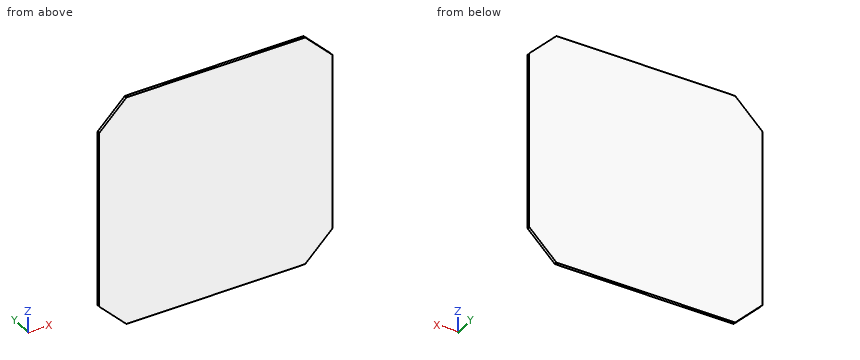
```python
from build123d import *

# Parameters (mm, degrees)
ESBO_O1_W                = 214
ESBO_O1_H                = 214
ESBO_O1_R                = 2.5
RESSALTO_EXTRUS_O1_DEPTH = 1.25
CHANFRO1_SIZE            = 25


with BuildPart() as part:
    # Esboço1 → Ressalto-extrusão1 (new, symmetric)
    with BuildSketch(Plane(origin=(0, 0, 0), x_dir=(1, 0, 0), z_dir=(0, 1, 0))):
        Rectangle(ESBO_O1_W, ESBO_O1_H)
        with Locations(Location((100, 100, 0), (0, 0, 270))):
            Circle(ESBO_O1_R, mode=Mode.SUBTRACT)
        with Locations(Location((-100, 100, 0), (0, 0, 90))):
            Circle(ESBO_O1_R, mode=Mode.SUBTRACT)
        with Locations(Location((100, -100, 0), (0, 0, 90))):
            Circle(ESBO_O1_R, mode=Mode.SUBTRACT)
        with Locations(Location((-100, -100, 0), (0, 0, 270))):
            Circle(ESBO_O1_R, mode=Mode.SUBTRACT)
    extrude(amount=RESSALTO_EXTRUS_O1_DEPTH, both=True)

    # Chanfro1
    chanfro1_edges = [part.edges().sort_by_distance(p)[0] for p in [
        (-107, 0, 107),
        (107, 0, 107),
        (107, 0, -107),
        (-107, 0, -107),
    ]]
    chamfer(chanfro1_edges, length=CHANFRO1_SIZE)


solid = part.part
```
CAD build for the part. Positions are in the model's coordinates, mm. Coordinates: 2 decimals unless noted, no trailing zeros. Write each loop counter-clockwise with the first axis right and the second up, starting at its lowest first coordinate (ties: lowest second). Pieces come first, ordered by that corner, then holes. Notation, with made-up numbers: (81, 24) -> (120, 24) arc R12 ccw to (120, 41) -> close; hole circle Ø2 at (-20.75, 44). An arc over 180 degrees is marked (long way). Return JSON: item names as keys, results as strings. Group by question number.
Q1. Drill centre lines: line 1 (Z direction, x = -92.5, y = 0.85); line 2 (X direction, y = 0.2, z = 93). Where is each one in solid material? Low to high.
Q2. Cut at A-A, the plane y = 0.15. Give the cut face in (x, z), then the cut area to 3 significant figures.
Q3. Cut at B-B, the plane z = 86.5. Give the cut face in (x, y), then the cut area to 4 significant figures.
Returned:
{
 "1": {"line 1": "z = -96.5 to 96.5", "line 2": "x = -96 to 96"},
 "2": {"outline": "(-107, -82) -> (-82, -107) -> (82, -107) -> (107, -82) -> (107, 82) -> (82, 107) -> (-82, 107) -> (-107, 82) -> close", "area": "44,500 mm2"},
 "3": {"outline": "(-102.5, -1.25) -> (102.5, -1.25) -> (102.5, 1.25) -> (-102.5, 1.25) -> close", "area": "512.5 mm2"}
}
